Read the model definition and answer for the solid it produces. Units are mm, in the model's axes. A direction names the side the tool comes from. Coordinates: 2 decimals unless noted, no trailing zeros. Order: outer loops, then holes, each group sorted by start corner. A loop starts at its lowest first (then second) coordinate and runs counter-clockwise, first axis right, second up. Notation, with made-up numbers: (48.5, -8) - (56.5, -8) arc R16 cw to (56.5, 22) - close; hole circle Ø5 at (7, 24). An arc over 180 degrees is marked (long way). Write item = value, one per line.
from build123d import *

# Parameters (mm, degrees)
F0_W     = 1.0496481662
F0_H     = 4.3377888929
F0_W_2   = 1.0251030326
F0_W_3   = 1.02070719
F0_W_4   = 1.0432768613
F0_W_5   = 1.0463846847
F0_W_6   = 1.0061389767
F0_W_7   = 1.0521755321
F0_W_8   = 1.0207062587
F0_W_9   = 1.0207053274
F0_W_10  = 1.0207034647
F0_W_11  = 0.9669847786
F0_W_12  = 1.0382413273
F1_DEPTH = 3.556
F0_W_13  = 5.6079216301
F0_W_14  = 5.9697218239
F0_W_15  = 5.3064189851
F0_W_16  = 5.8491192758
F0_W_17  = 6.1098765582
F0_W_18  = 5.6421123445
F0_W_19  = 5.6237019598
F0_W_20  = 6.3587981276
F0_W_21  = 6.3517062808
F0_W_22  = 6.2316799886
F0_W_23  = 6.3391225412
F0_W_24  = 5.909351632
F0_W_25  = 5.6944675744
F0_W_26  = 5.9630740434
F0_W_27  = 5.640745163
F0_W_28  = 5.8556310833
F0_W_29  = 5.5870227516
F0_W_30  = 5.0498098135
F0_W_31  = 5.963075906
F2_DEPTH = 2.032


with BuildPart() as f1:
    # F0 (on Front) → F1 (new body)
    with BuildSketch(Plane.XZ):
        with Locations((-68.5631759169, -0.3711055536)):
            Rectangle(F0_W, F0_H)
        Polygon((69.088, 1.7977888929), (69.088, 2.54), (-69.088, 2.54), (-69.088, 1.7977888929), (-68.0383518338, 1.7977888929), (-62.4304302037, 1.7977888929), (-61.4053271711, 1.7977888929), (-55.4356053472, 1.7977888929), (-54.4105023146, 1.7977888929), (-49.1040833294, 1.7977888929), (-48.0789802969, 1.7977888929), (-42.229861021, 1.7977888929), (-41.2047579885, 1.7977888929), (-35.5968363583, 1.7977888929), (-34.5717333257, 1.7977888929), (-28.4618567675, 1.7977888929), (-27.4411495775, 1.7977888929), (-21.799037233, 1.7977888929), (-20.7557603717, 1.7977888929), (-15.1320584118, 1.7977888929), (-14.0856737271, 1.7977888929), (-7.7268755995, 1.7977888929), (-6.7207366228, 1.7977888929), (-0.369030342, 1.7977888929), (0.6831451901, 1.7977888929), (6.9148251787, 1.7977888929), (7.9355314374, 1.7977888929), (14.2746539786, 1.7977888929), (15.2953602374, 1.7977888929), (21.2047118694, 1.7977888929), (22.2254171968, 1.7977888929), (27.9198847711, 1.7977888929), (28.9405900985, 1.7977888929), (34.9036641419, 1.7977888929), (35.9243713319, 1.7977888929), (41.5651164949, 1.7977888929), (42.5858236849, 1.7977888929), (48.4414547682, 1.7977888929), (49.4621582329, 1.7977888929), (55.0491809845, 1.7977888929), (56.0698881745, 1.7977888929), (61.119697988, 1.7977888929), (62.0866827667, 1.7977888929), (68.0497586727, 1.7977888929), align=None)
        with Locations((-61.9178786874, -0.3711055536)):
            Rectangle(F0_W_2, F0_H)
        with Locations((-54.9230538309, -0.3711055536)):
            Rectangle(F0_W_2, F0_H)
        with Locations((-48.5915318131, -0.3711055536)):
            Rectangle(F0_W_2, F0_H)
        with Locations((-41.7173095047, -0.3711055536)):
            Rectangle(F0_W_2, F0_H)
        with Locations((-35.084284842, -0.3711055536)):
            Rectangle(F0_W_2, F0_H)
        with Locations((-27.9515031725, -0.3711055536)):
            Rectangle(F0_W_3, F0_H)
        with Locations((-21.2773988023, -0.3711055536)):
            Rectangle(F0_W_4, F0_H)
        with Locations((-14.6088660695, -0.3711055536)):
            Rectangle(F0_W_5, F0_H)
        with Locations((-7.2238061111, -0.3711055536)):
            Rectangle(F0_W_6, F0_H)
        with Locations((0.1570574241, -0.3711055536)):
            Rectangle(F0_W_7, F0_H)
        with Locations((7.425178308, -0.3711055536)):
            Rectangle(F0_W_8, F0_H)
        with Locations((14.785007108, -0.3711055536)):
            Rectangle(F0_W_8, F0_H)
        with Locations((21.7150645331, -0.3711055536)):
            Rectangle(F0_W_9, F0_H)
        with Locations((28.4302374348, -0.3711055536)):
            Rectangle(F0_W_9, F0_H)
        with Locations((35.4140177369, -0.3711055536)):
            Rectangle(F0_W_3, F0_H)
        with Locations((42.0754700899, -0.3711055536)):
            Rectangle(F0_W_3, F0_H)
        with Locations((48.9518065006, -0.3711055536)):
            Rectangle(F0_W_10, F0_H)
        with Locations((55.5595345795, -0.3711055536)):
            Rectangle(F0_W_3, F0_H)
        with Locations((61.6031903774, -0.3711055536)):
            Rectangle(F0_W_11, F0_H)
        with Locations((68.5688793364, -0.3711055536)):
            Rectangle(F0_W_12, F0_H)
    extrude(amount=F1_DEPTH)

    # F0 (on Front) → F2 (join)
    with BuildSketch(Plane.XZ):
        with Locations((-65.2343910187, -0.3711055536)):
            Rectangle(F0_W_13, F0_H)
        with Locations((-58.4204662591, -0.3711055536)):
            Rectangle(F0_W_14, F0_H)
        with Locations((-51.757292822, -0.3711055536)):
            Rectangle(F0_W_15, F0_H)
        with Locations((-45.1544206589, -0.3711055536)):
            Rectangle(F0_W_16, F0_H)
        with Locations((-38.4007971734, -0.3711055536)):
            Rectangle(F0_W_13, F0_H)
        with Locations((-31.5167950466, -0.3711055536)):
            Rectangle(F0_W_17, F0_H)
        with Locations((-24.6200934052, -0.3711055536)):
            Rectangle(F0_W_18, F0_H)
        with Locations((-17.9439093918, -0.3711055536)):
            Rectangle(F0_W_19, F0_H)
        with Locations((-10.9062746633, -0.3711055536)):
            Rectangle(F0_W_20, F0_H)
        with Locations((-3.5448834824, -0.3711055536)):
            Rectangle(F0_W_21, F0_H)
        with Locations((3.7989851844, -0.3711055536)):
            Rectangle(F0_W_22, F0_H)
        with Locations((11.105092708, -0.3711055536)):
            Rectangle(F0_W_23, F0_H)
        with Locations((18.2500360534, -0.3711055536)):
            Rectangle(F0_W_24, F0_H)
        with Locations((25.0726509839, -0.3711055536)):
            Rectangle(F0_W_25, F0_H)
        with Locations((31.9221271202, -0.3711055536)):
            Rectangle(F0_W_26, F0_H)
        with Locations((38.7447439134, -0.3711055536)):
            Rectangle(F0_W_27, F0_H)
        with Locations((45.5136392266, -0.3711055536)):
            Rectangle(F0_W_28, F0_H)
        with Locations((52.2556696087, -0.3711055536)):
            Rectangle(F0_W_29, F0_H)
        with Locations((58.5947930813, -0.3711055536)):
            Rectangle(F0_W_30, F0_H)
        with Locations((65.0682207197, -0.3711055536)):
            Rectangle(F0_W_31, F0_H)
    extrude(amount=F2_DEPTH)


solid = f1.part
1) Straight lines are drawn through the part: line 1 along Y through (x, z) = (17.5, -2); line 2 along Z through (x, y) = (20.5, -2.2). For each, find the intervals that lie inside material, in ascending order. Write a range as from..to.
Returned:
line_1 = -2.03..0
line_2 = 1.8..2.54
2) The part is cut by section A-A (x = 19). Determine the outline of the cut face in (y, z), and give its area (3 significant figures).
Returned:
outline = (-3.56, 1.8) - (-2.03, 1.8) - (-2.03, -2.54) - (0, -2.54) - (0, 2.54) - (-3.56, 2.54) - close
area = 11.5 mm^2
3) For faces 1 (the face through (-58, -2.032, 0)), 2 (the face through (-1, 0, 0)), determine the directions among +Z, -Z, +X, -X, +Y, -Y from which every point of the face is accessible in a straight line to the end or side of a thin tool.
Returned:
face_1 = -Z, -Y
face_2 = +Z, -Z, +X, -X, +Y
4) Determine the mould class of faces 3 (the face through (69.088, -2, 0)), 4 (the face through (4, -2.032, 0)), 5 (the face through (-1, -1, -2.54)) for opening direction X: pulls with the +X half, pulls with the -X half, needs draft (parallel to the pull), parting line crosses it, or undercut.
Returned:
face_3 = pulls with the +X half
face_4 = undercut
face_5 = needs draft
5) Flat-ended cylindrical pins translate along their axes: pin 1 Ø2 at (x, z) = (11.5, -1.5) entering from -Y; pin 2 Ø3 at (x, z) = (-43.5, 1) entering from +Y; pin 3 Ø0.8 at (x, y) = (53, -3) entering from -Z. Find the tip coordinate at first contact, or state that the pin passes through.
Returned:
pin_1 = -2.03
pin_2 = 0
pin_3 = 1.8
